Autodesk Inventor part; units mm, degrees
ref_plane "YZ Plane" through (0, 0, 0) normal (1, 0, 0) x (0, 1, 0)
ref_plane "XZ Plane" through (0, 0, 0) normal (0, 1, 0) x (-1, 0, 0)
ref_plane "XY Plane" through (0, 0, 0) normal (0, 0, 1) x (1, 0, 0)
sketch "Sketch1" plane through (0, 0, 0) normal (0, 1, 0) x (-1, 0, 0)
  line L0 (52, 58.6471) -> (-48, 58.6471)
  line L1 (-48, 58.6471) -> (-48, -16.3529)
  line L2 (-48, -16.3529) -> (52, -16.3529)
  line L3 (52, -16.3529) -> (52, 58.6471)
  point P0 (0, 0)
  dimension "d0" = 100
  dimension "d1" = 75
extrude "Extrusion1" add sketch "Sketch1" along normal blind 60
sketch "Sketch2" plane through (0, 60, 0) normal (0, 1, 0) x (1, 0, 0)
  line L0 (-47, -53.6471) -> (43, -53.6471)
  line L1 (43, -53.6471) -> (43, 11.3529)
  line L2 (43, 11.3529) -> (-47, 11.3529)
  line L3 (-47, 11.3529) -> (-47, -53.6471)
  line L4 (-52, 16.3529) -> (-52, -58.6471)
  line L5 (-52, -58.6471) -> (48, -58.6471)
  line L6 (48, 16.3529) -> (-52, 16.3529)
  line L7 (48, -58.6471) -> (48, 16.3529)
  point P0 (0, 0)
  dimension "d4" = 5
  dimension "d5" = 5
  dimension "d6" = 5
  dimension "d7" = 5
extrude "Extrusion2" cut sketch "Sketch2" against normal blind 59 contours L3 L2 L1 L0
sketch "Sketch3" plane through (48, 0, -16.3529) normal (0, 0, -1) x (-1, 0, 0)
  circle A0 centre (48, 60) radius 13
  point P0 (48, 0)
  dimension "d10" = 26
  dimension "d11" = 60
sketch "Sketch13" plane through (0, 1, 0) normal (0, 1, 0) x (1, 0, 0)
  line L0 (-47, -53.6471) -> (-47, 11.3529)
  line L1 (43, 11.3529) -> (43, -53.6471)
  line L2 (-47, 11.3529) -> (43, 11.3529)
  line L3 (43, 11.3529) -> (43, -13.6471)
  line L4 (43, -13.6471) -> (-47, -13.6471)
  line L5 (-47, -13.6471) -> (-47, 11.3529)
  point P0 (0, 0)
  dimension "d44" = 25
extrude "Extrusion14" add sketch "Sketch13" along normal blind 59
sketch "Sketch14" plane through (-47, 1, 13.6471) normal (0, 0, 1) x (1, 0, 0)
  line L0 (0, 59) -> (90, 59)
  circle A0 centre (47, 59) radius 23.505
  point P0 (47, -1)
  dimension "d47" = 47.01
extrude "Extrusion15" cut sketch "Sketch14" against normal blind 12.1
sketch "Sketch15" plane through (0, 1, 0) normal (0, 1, 0) x (1, 0, 0)
  line L0 (-47, -53.6471) -> (-47, -13.6471)
  line L1 (43, -13.6471) -> (43, -53.6471)
  line L2 (-47, -53.6471) -> (43, -53.6471)
  line L3 (43, -53.6471) -> (43, -28.6471)
  line L4 (43, -28.6471) -> (-47, -28.6471)
  line L5 (-47, -28.6471) -> (-47, -53.6471)
  point P0 (0, 0)
  point P1 (-47, -28.6471)
  dimension "d50" = 25
extrude "Extrusion16" add sketch "Sketch15" along normal blind 59
sketch "Sketch16" plane through (43, 1, 28.6471) normal (0, 0, -1) x (-1, 0, 0)
  line L0 (0, 59) -> (90, 59)
  circle A0 centre (43, 59) radius 23.505
  point P0 (43, -1)
  dimension "d53" = 47.01
extrude "Extrusion17" cut sketch "Sketch16" against normal blind 12.1
sketch "Sketch17" plane through (0, 1, 0) normal (0, 1, 0) x (1, 0, 0)
  line L0 (23.505, -13.6471) -> (43, -13.6471)
  line L1 (-47, -28.6471) -> (43, -28.6471)
  line L2 (43, -28.6471) -> (43, -13.6471)
  line L3 (43, -13.6471) -> (-47, -13.6471)
  line L4 (-47, -13.6471) -> (-47, -28.6471)
  point P0 (0, 0)
extrude "Extrusion18" add sketch "Sketch17" along normal blind 59
extrude "Extrusion19" cut sketch "Sketch3" against normal blind 75
sketch "Sketch19" plane through (0, 0, 0) normal (0, -1, 0) x (1, 0, 0)
  line L0 (48, 58.6471) -> (48, -16.3529)
  line L1 (-52, -16.3529) -> (-52, 58.6471)
  line L2 (48, 58.6471) -> (-52, 58.6471)
  line L3 (-52, 58.6471) -> (-52, -16.3529)
  line L4 (-52, -16.3529) -> (48, -16.3529)
  line L5 (48, -16.3529) -> (48, 58.6471)
  point P0 (0, 0)
extrude "Extrusion21" add sketch "Sketch19" along normal blind 30
sketch "Sketch20" plane through (0, -30, 0) normal (0, -1, 0) x (1, 0, 0)
  point P0 (0, 0)
sketch "Sketch21" plane through (0, -30, 0) normal (0, -1, 0) x (1, 0, 0)
  line L0 (23, -3.8529) -> (-27, -3.8529)
  line L1 (-27, -3.8529) -> (-27, 46.1471)
  line L2 (-27, 46.1471) -> (23, 46.1471)
  line L3 (23, 46.1471) -> (23, -3.8529)
  line L4 (-52, -16.3529) -> (48, -16.3529)
  line L5 (48, 58.6471) -> (-52, 58.6471)
  line L6 (-52, 58.6471) -> (-52, -16.3529)
  line L7 (48, -16.3529) -> (48, 58.6471)
  point P0 (0, 0)
  dimension "d66" = 12.5
  dimension "d67" = 12.5
  dimension "d68" = 25
  dimension "d69" = 25
extrude "Extrusion22" add sketch "Sketch21" along normal blind 30 contours L0 L1 L2 L3
sketch "Sketch22" plane through (0, -60, 0) normal (0, -1, 0) x (1, 0, 0)
  line L0 (48, -28.8529) -> (-52, -28.8529)
  line L1 (-52, -28.8529) -> (-52, 71.1471)
  line L2 (-52, 71.1471) -> (48, 71.1471)
  line L3 (48, 71.1471) -> (48, -28.8529)
  line L4 (-27, -3.8529) -> (23, -3.8529)
  line L5 (23, -3.8529) -> (23, 46.1471)
  line L6 (23, 46.1471) -> (-27, 46.1471)
  line L7 (-27, 46.1471) -> (-27, -3.8529)
  point P0 (0, 0)
  dimension "d72" = 25
  dimension "d73" = 25
  dimension "d74" = 25
  dimension "d75" = 25
extrude "Extrusion23" add sketch "Sketch22" along normal blind 20 contours L0 L1 L2 L3 | L7 L6 L5 L4
equation "\"d6\" = d5"
equation "\"d7\" = d4"
equation "\"d67\" = d66"
equation "\"d68\" = d69"
equation "\"d72\" = d73"
equation "\"d74\" = d73"
equation "\"d75\" = d73"
properties part number "casing bottom"
Geometry: final body of the model. Coordinates: model frame, mm. A direction names the side the tool comes from. Coordinates: 2 decimals unless noted, no trailing zeros. Order: outer loops, then holes, each group sorted by start corner. A loop starts at its lowest first (then second) coordinate and runs counter-clockwise, first axis right, second up. Notation, with made-up numbers: (67, 82.5) -> (106, 82.5) arc R21 ccw to (106, 102.5) -> close; hole circle Ø9 at (-8, 80.25). An arc over 180 degrees is marked (long way). Answer in a Markdown table with one row per item.
Item 1: Section C-C on y = 50.5. Output: boundary loops of the cut face in (x, z), plus the area to 3 significant figures.
Return value:
| item | result |
|---|---|
| outline | (-52, -16.35) -> (-8.87, -16.35) -> (-8.87, 1.55) -> (-21.5, 1.55) -> (-21.5, 13.65) -> (-8.87, 13.65) -> (-8.87, 28.65) -> (-21.5, 28.65) -> (-21.5, 40.75) -> (-8.87, 40.75) -> (-8.87, 58.65) -> (-52, 58.65) -> close; (8.87, -16.35) -> (48, -16.35) -> (48, 58.65) -> (8.87, 58.65) -> (8.87, 40.75) -> (21.5, 40.75) -> (21.5, 28.65) -> (8.87, 28.65) -> (8.87, 13.65) -> (21.5, 13.65) -> (21.5, 1.55) -> (8.87, 1.55) -> close |
| area | 5,560 mm² |
Item 2: Contact query for flat-ended pins moving along their axis: P1, Ø7, axis at x = -9.5, y = 47, coming from the +Z side; P2, Ø1, axis at y = -41, z = 27, coming from the +X side; P3, Ø12, axis at x = -36, y = -32, coming from the -Z side. Output: stop coordinate, or through.
Return value:
| item | result |
|---|---|
| P1 | stops at z = 58.65 |
| P2 | stops at x = 23 |
| P3 | stops at z = -16.35 |
Item 3: Ray query, L1, parallel to Z at x = -19, y = 50; L2, parallel to Y at x = 37, z = 44; L3, parallel to Z at x = 20, y = 35. Return the intervals inside material, ascending.
Return value:
| item | result |
|---|---|
| L1 | z = -16.35 to 1.55, 13.65 to 28.65, 40.75 to 58.65 |
| L2 | y = -80 to -60, -30 to 60 |
| L3 | z = -16.35 to 58.65 |
Item 4: Section A-A on x = 31.5. Output: boundary loops of the cut face in (y, z).
Return value:
| item | result |
|---|---|
| outline | (-80, -28.85) -> (-60, -28.85) -> (-60, 71.15) -> (-80, 71.15) -> close; (-30, -16.35) -> (60, -16.35) -> (60, 58.65) -> (-30, 58.65) -> close |
Item 5: Section D-D on x = 0. Output: boundary loops of the cut face in (y, z) (3 decimals), plus the area to 3 significant figures.
Return value:
| item | result |
|---|---|
| outline | (-80, -28.853) -> (-60, -28.853) -> (-60, -3.853) -> (-30, -3.853) -> (-30, -16.353) -> (47, -16.353) -> (47, 1.547) -> (36.495, 1.547) -> (36.495, 13.647) -> (47, 13.647) -> (47, 28.647) -> (36.495, 28.647) -> (36.495, 40.747) -> (47, 40.747) -> (47, 58.647) -> (-30, 58.647) -> (-30, 46.147) -> (-60, 46.147) -> (-60, 71.147) -> (-80, 71.147) -> close |
| area | 9,020 mm² |
Item 6: Access query for faces 4 (the flat face through (-36, -60, 22)), 5 (the flat face through (-2, -45, -3.853)), 6 (the flat face through (23, -45, 21)), 7 (the flat face through (0, 45, 13.647)), 8 (the flat face through (-3, 16, -16.353)). Directions: +Z, -Z, +X, -X, +Y, -Y. A direction counts if a zero-diameter tool reaches every point of the face in a straight line with its end or side. Return the directions, or none.
Return value:
| item | result |
|---|---|
| face 4 | none |
| face 5 | -Z, +X, -X |
| face 6 | +Z, -Z, +X |
| face 7 | +Y |
| face 8 | -Z, +X, -X, +Y |
Item 7: Draft query along Y for faces 1 (the cylindrical face through (0.5, 36.5, 34.6)), 2 (the flat face through (-2, -45, 46.147)), 3 (the flat face through (0, 46, 1.547)). Return one class per face: released by +Y, released by -Y, zero draft, split by the parting line, or undercut.
Return value:
| item | result |
|---|---|
| face 1 | released by +Y |
| face 2 | undercut |
| face 3 | zero draft |
Item 8: Section B-B on z = 49. Output: boundary loops of the cut face in (x, y).
Return value:
| item | result |
|---|---|
| outline | (-52, -80) -> (48, -80) -> (48, -60) -> (-52, -60) -> close; (-52, -30) -> (48, -30) -> (48, 60) -> (13, 60) arc R13 cw to (-13, 60) -> (-52, 60) -> close |
